Can you work these out from the model? Positions are in its coordinate system, mm. Face numbers are marked on the shaded views. A direction names the side the tool comes from. Coordinates: 2 decimals unless noted, no trailing zeros. Loops run counter-clockwise (first coordinate to the right, second up) from the corner with the lowest first, then second, coordinate; pieces in that order, holes last. Notation, with made-up numbers: (73, 72.25) -> (123, 72.25) arc R25 cw to (123, 101.25) -> close; hole circle Ø11 at (49, -19). An arc over 180 degrees is marked (long way). Use one line per item in the form item = value. Start each with the question number.
(1) I need wall thicknesses on line 1 (Z direction, x = -2, y = -2.25); line 2 (Z direction, x = 9.25, y = 4.5); line 3 (Y direction, x = 15, z = -7.9). Which ranges of each line are inside material? Lowest first, please. Write a range as [from, to].
(2) Imagine slicing it at A-A (z = -8). List the corners of the cut face in (x, y) for me.
(3) Imagine slicing it at D-D (z = -28). List the corners of the cut face in (x, y) for me.
(4) Thinking about a two-plate mould opening in Z: for the marked faces 6, 7 and 8, which applies, released by +Z, released by -Z, zero draft, split by the parting line, or undercut?
(5) Imagine slicing it at B-B (y = 4). List the corners of the cut face in (x, z) for me.
(6) Imagine slicing it at C-C (y = -1.5). List the corners of the cut face in (x, z) for me, plus the area to 3 significant figures.
(7) On a 3-axis mill with a long thin cutter (end or side, diameter ignored), from which of +Z, -Z, +X, -X, +Y, -Y can I reach the whole of each face in a straight line? I mean the marked faces 1, 2, 3, 4 and 5. Say none if no direction works.
(8) I'm going to push flat-ended pins straight in: pin 1 (3 mm diameter, centred on x = 11, y = 2.5, fed in from +Z); pin 2 (11.5 mm diameter, centred on x = -2.5, z = -10.5, fed in from +Y); pin 3 (3 mm diameter, centred on y = -1, z = -19, fed in from +X). Where does each tip first touch, or does it pass through?
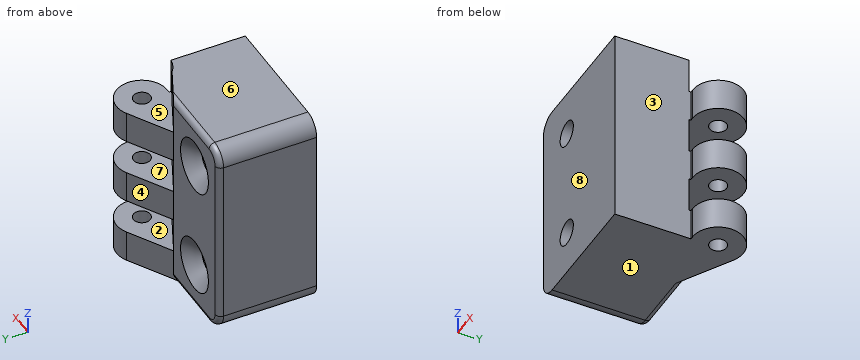
```python
from build123d import *

# Parameters (mm, degrees)
CROQUIS1_R              = 1.5
SALIENTE_EXTRUIR1_DEPTH = 36
CORTAR_EXTRUIR1_DEPTH   = 6.3
MATRIZL1_COUNT          = 3
MATRIZL1_PITCH          = 12
CROQUIS3_R              = 2.25
CORTAR_EXTRUIR2_DEPTH   = 8.5
CHAFL_N1_SIZE           = 2.5
REDONDEO1_R             = 3
REDONDEO2_R             = 1
SKETCH1_R               = 2.25
BOSS_EXTRUDE2_DEPTH     = 10


with BuildPart() as part:
    # Croquis1 → Saliente-Extruir1 (new body)
    with BuildSketch(Plane.XY):
        with BuildLine():
            Line((12.75, 7.897114317), (5.133974596, 3.5))
            Line((5.133974596, 3.5), (-10, 3.5))
            Line((-10, 3.5), (-10, -4))
            Line((-10, -4), (14.4, -4))
            Line((14.4, -4), (14.4, -0.5))
            Line((14.4, -0.5), (15, -0.5))
            ThreePointArc((15, -0.5), (19.346666218, 5.164685703), (12.75, 7.897114317))
        make_face()
        with Locations((15, 4)):
            Circle(CROQUIS1_R, mode=Mode.SUBTRACT)
    extrude(amount=-SALIENTE_EXTRUIR1_DEPTH)

    # Croquis2 → Cortar-Extruir1 (cut)
    with BuildSketch(Plane.XY):
        with BuildLine():
            Line((14.4, -0.842600764), (15, -0.5))
            ThreePointArc((15, -0.5), (19.346666218, 5.164685703), (12.75, 7.897114317))
            Line((12.75, 7.897114317), (5.133974596, 3.5))
            Line((5.133974596, 3.5), (11.80761005, 0.309549003))
            ThreePointArc((11.80761005, 0.309549003), (13.018228657, -0.459076642), (14.4, -0.842600764))
        make_face()
    cortar_extruir1 = extrude(amount=-CORTAR_EXTRUIR1_DEPTH, mode=Mode.SUBTRACT)

    # MatrizL1: Cortar-Extruir1 ×3
    with Locations(*[(0, 0, -i * MATRIZL1_PITCH) for i in range(1, MATRIZL1_COUNT)]):
        add(cortar_extruir1, mode=Mode.SUBTRACT)

    # Croquis3 → Cortar-Extruir2 (cut, through all)
    with BuildSketch(Plane(origin=(0, 3.5, 0), x_dir=(1, 0, 0), z_dir=(0, 1, 0))):
        with Locations((-2, 28)):
            Circle(CROQUIS3_R)
        with Locations((-2, 8)):
            Circle(CROQUIS3_R)
    extrude(amount=-CORTAR_EXTRUIR2_DEPTH, mode=Mode.SUBTRACT)

    # Chaflán1
    chafl_n1_edges = [part.edges().sort_by_distance(p)[0] for p in [
        (-4.25, 3.5, -28),
        (-4.25, 3.5, -8),
    ]]
    chamfer(chafl_n1_edges, length=CHAFL_N1_SIZE)

    # Redondeo1
    redondeo1_edges = [part.edges().sort_by_distance(p)[0] for p in [
        (-10, -0.25, -36),
        (-10, -0.25, 0),
    ]]
    fillet(redondeo1_edges, radius=REDONDEO1_R)

    # Redondeo2
    redondeo2_edges = [part.edges().sort_by_distance(p)[0] for p in [
        (-10, 3.5, -18),
        (-9.121320344, 3.5, -0.878679656),
        (-9.121320344, 3.5, -35.121320344),
        (-0.933012702, 3.5, -36),
        (-0.933012702, 3.5, 0),
    ]]
    fillet(redondeo2_edges, radius=REDONDEO2_R)

    # Sketch1 → Boss-Extrude2 (add)
    with BuildSketch(Plane.XZ.offset(4)):
        with BuildLine():
            Line((-10, -3), (-10, -33))
            ThreePointArc((-10, -33), (-9.121320344, -35.121320344), (-7, -36))
            Line((-7, -36), (14.4, -36))
            Line((14.4, -36), (14.4, 0))
            Line((14.4, 0), (-7, 0))
            ThreePointArc((-7, 0), (-9.121320344, -0.878679656), (-10, -3))
        make_face()
        with Locations((-2, -8)):
            Circle(SKETCH1_R, mode=Mode.SUBTRACT)
        with Locations((-2, -28)):
            Circle(SKETCH1_R, mode=Mode.SUBTRACT)
    extrude(amount=BOSS_EXTRUDE2_DEPTH)


solid = part.part
```
Worked out:
q1.line_1 = [-36, -30.25], [-25.75, -10.25], [-5.75, 0]
q1.line_2 = [-36, -30.3], [-24, -18.3], [-12, -6.3]
q1.line_3 = [-0.5, 2.5], [5.5, 8.5]
q2.outline = (-10, -14) -> (-4.25, -14) -> (-4.25, 1) -> (-6.75, 3.5) -> (-9, 3.5) arc R1 ccw to (-10, 2.5) -> close; (0.25, -14) -> (14.4, -14) -> (14.4, -0.5) -> (15, -0.5) arc R4.5 ccw (long way) to (12.75, 7.9) -> (5.13, 3.5) -> (2.75, 3.5) -> (0.25, 1) -> close; hole circle Ø3 at (15, 4)
q3.outline = (-10, -14) -> (-4.25, -14) -> (-4.25, 1) -> (-6.75, 3.5) -> (-9, 3.5) arc R1 ccw to (-10, 2.5) -> close; (0.25, -14) -> (14.4, -14) -> (14.4, -0.84) arc R4.88 cw to (11.81, 0.31) -> (5.13, 3.5) -> (2.75, 3.5) -> (0.25, 1) -> close
q4.face_6 = released by +Z
q4.face_7 = undercut
q4.face_8 = zero draft
q5.outline = (6, -36) -> (13.5, -36) -> (13.5, -30.3) -> (6, -30.3) -> close; (6, -24) -> (13.5, -24) -> (13.5, -18.3) -> (6, -18.3) -> close; (6, -12) -> (13.5, -12) -> (13.5, -6.3) -> (6, -6.3) -> close; (16.5, -36) -> (19.5, -36) -> (19.5, -30.3) -> (16.5, -30.3) -> close; (16.5, -24) -> (19.5, -24) -> (19.5, -18.3) -> (16.5, -18.3) -> close; (16.5, -12) -> (19.5, -12) -> (19.5, -6.3) -> (16.5, -6.3) -> close
q6.outline = (-10, -33) arc R3 ccw to (-7, -36) -> (14.4, -36) -> (14.4, 0) -> (-7, 0) arc R3 ccw to (-10, -3) -> close; hole circle Ø4.5 at (-2, -28); hole circle Ø4.5 at (-2, -8)
q6.area = 843 mm2
q7.face_1 = -Z, +X, -X, +Y, -Y
q7.face_2 = +X, +Y
q7.face_3 = +Z, -Z, +X, -Y
q7.face_4 = +Z, -Z, -X, +Y
q7.face_5 = +Z, +X, +Y
q8.pin_1 = -6.3
q8.pin_2 = 3.5
q8.pin_3 = 17.83
